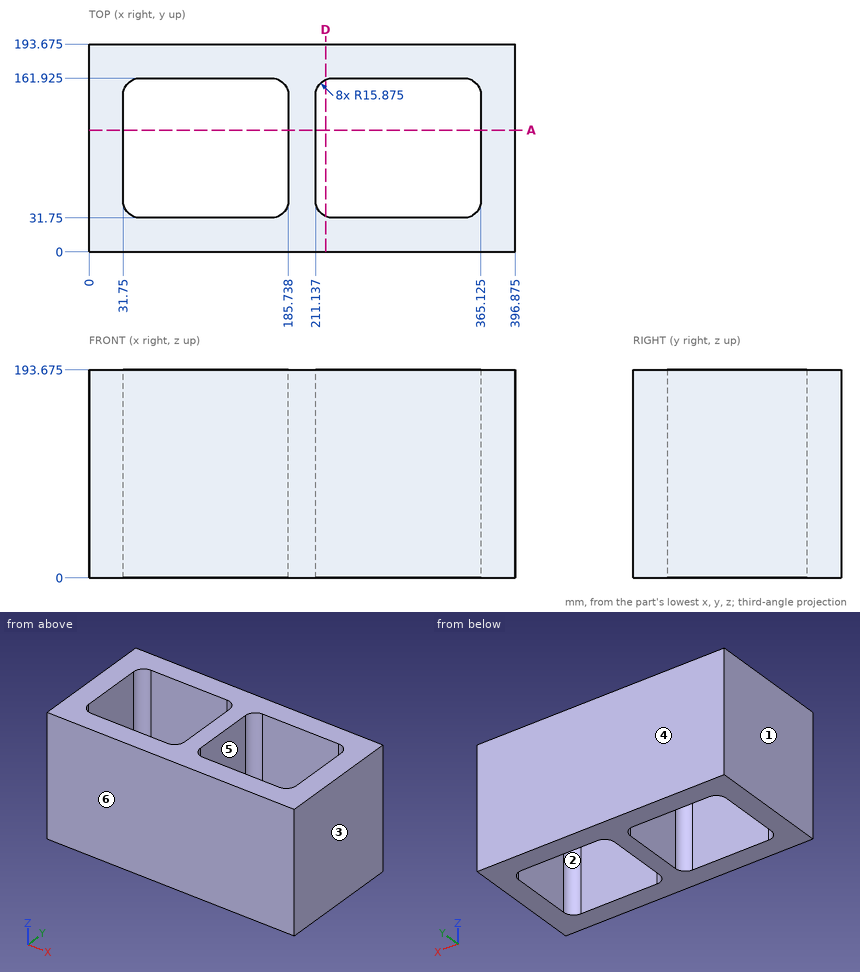
Check sheet for the drawn part. Datum: minimum x, y, z corner. Units: mm. A direction names the side the tool comes from. Give positions to 0.01 mm unless a question says otherwise; leave off trailing zeros. Order: outer loops, then holes, each group sorted by start corner. A loop starts at its lowest first (then second) coordinate and runs counter-clockwise, first axis right, second up. Notation, with made-up numbers: (85.25, 46.25) -> (113.25, 46.25) arc R21 ccw to (113.25, 82.25) -> close; hole circle Ø11 at (61.5, -32). An arc over 180 degrees is marked (long way). Use a Markdown table: item, result.
1) Material ranges on probe 1 along Y at (x, z) = (46, 146) (1 decimal); probe 2 along X at (y, z) = (158, 48) (1 decimal); probe 3 along X at (y, z) = (39.5, 146) (1 decimal), recorded low to high.
Results:
| item | result |
|---|---|
| probe 1 | 0 to 31.8, 161.8 to 193.7 |
| probe 2 | 0 to 37.2, 180.3 to 216.6, 359.7 to 396.9 |
| probe 3 | 0 to 34, 183.5 to 213.4, 362.9 to 396.9 |
2) Tool access check on the marked faces 5 and 6. Record the directions out of +Z, -Z, +X, -X, +Y, -Y that give a thin tool (end or side, any length) a straight path to the whole face; none if there is none.
Results:
| item | result |
|---|---|
| face 5 | +Z, -Z |
| face 6 | +Z, -Z, +X, -X, -Y |
3) Section check D-D, the plane x = 220.5. Record the boundary of the cut face in (y, z) (1 decimal).
Results:
| item | result |
|---|---|
| outline | (0, 0) -> (33.1, 0) -> (33.1, 193.7) -> (0, 193.7) -> close; (160.5, 0) -> (193.7, 0) -> (193.7, 193.7) -> (160.5, 193.7) -> close |
4) Section check A-A, the plane y = 113.5. Give the number of separate pieces and of enclosed holes in the cut face, then the cut area to 3 significant figures.
Results:
| item | result |
|---|---|
| separate pieces | 3 |
| enclosed holes | 0 |
| area | 17,200 mm² |
5) Mould release check, pull along X, two halves, no side actions. Record for the marked faces 1, 2, 3 and 4: pulls with the +X half, pulls with the -X half, needs draft (parallel to the pull), parting line crosses it, or undercut.
Results:
| item | result |
|---|---|
| face 1 | pulls with the -X half |
| face 2 | undercut |
| face 3 | pulls with the +X half |
| face 4 | needs draft |
6) Depth check by flat-ended pin: pin 1 Ø1 at (x, y) = (293, 33) entering from -Z. Enter the tip coordinate at first touch or a pass-through.
Results:
| item | result |
|---|---|
| pin 1 | through |
